Study the drawing (mm; zero at the part's minimum x, y, z) and answer. A direction names the side the tool comes from. Coordinates: 2 decimals unless noted, no trailing zeros. Order: outer loops, then holes, each group sorted by start corner. A loop starts at its lowest first (then second) coordinate and runs counter-clockwise, first axis right, second up. Notation, with made-up numbers: (8, 79) -> (19, 79) arc R32 ccw to (19, 105) -> close; hole circle Ø5 at (-11.75, 86). An arc over 180 degrees is marked (long way). Answer in a Markdown table with one row per item. Add a question column.
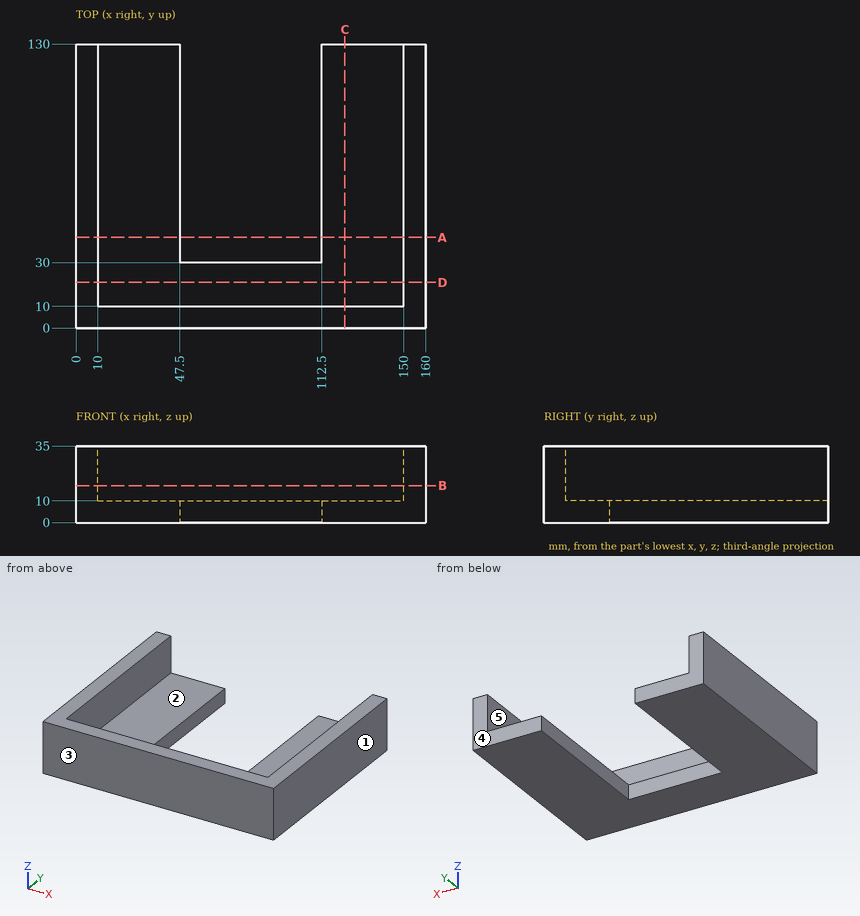
Q1. Determine the mould class of the marked faces 1, 2 and 3 for opening direction X: +X half, -X half, draft (parallel to the pull), parting line (faces both ways), or undercut.
Q2. For the marked faces 4 and 5, determine the directions among +Z, -Z, +X, -X, +Y, -Y from which every point of the face is accessible in a straight line to the end or side of a thin tool.
Q3. A cutting plane is placed at B-B (z = 17). Determine the outline of the cut face in (x, y), then the cut area to 3 significant figures.
Q4. Given pin 1 (12.5 mm diameter, centred on x = 52, z = 25.5, fed in from +Y); pin 2 (5 mm diameter, centred on x = 78, z = 7, fed in from +Y); pin 3 (12 mm diameter, centred on x = 132, y = 44.5, fed in from +Z), each flat-ended and moving along its own axis, determine where each tip first touches the part or whether it passes through.
Q5. A cutting plane is placed at D-D (y = 21). Determine the outline of the cut face in (x, z).
Q6. Straight lines are drawn through the part: line 1 (X direction, y = 29.5, z = 15); line 2 (X direction, y = 99.5, z = 4.5); line 3 (Y direction, x = 102, z = 32). For each, find the intervals that lie inside material, in ascending order.
Q7. A cutting plane is placed at A-A (y = 41.5). Determine the outline of the cut face in (x, z).
Q8. A cutting plane is placed at C-C (x = 123). Determine the outline of the cut face in (y, z).
Returned:
| question | item | result |
|---|---|---|
| 1 | face 1 | +X half |
| 1 | face 2 | undercut |
| 1 | face 3 | draft |
| 2 | face 4 | +Z, -Z, +X, -X, +Y |
| 2 | face 5 | +Z, +Y |
| 3 | outline | (0, 0) -> (160, 0) -> (160, 130) -> (150, 130) -> (150, 10) -> (10, 10) -> (10, 130) -> (0, 130) -> close |
| 3 | area | 4,000 mm² |
| 4 | pin 1 | stops at y = 10 |
| 4 | pin 2 | stops at y = 30 |
| 4 | pin 3 | stops at z = 10 |
| 5 | outline | (0, 0) -> (160, 0) -> (160, 35) -> (150, 35) -> (150, 10) -> (10, 10) -> (10, 35) -> (0, 35) -> close |
| 6 | line 1 | x = 0 to 10, 150 to 160 |
| 6 | line 2 | x = 0 to 47.5, 112.5 to 160 |
| 6 | line 3 | y = 0 to 10 |
| 7 | outline | (0, 0) -> (47.5, 0) -> (47.5, 10) -> (10, 10) -> (10, 35) -> (0, 35) -> close; (112.5, 0) -> (160, 0) -> (160, 35) -> (150, 35) -> (150, 10) -> (112.5, 10) -> close |
| 8 | outline | (0, 0) -> (130, 0) -> (130, 10) -> (10, 10) -> (10, 35) -> (0, 35) -> close |
